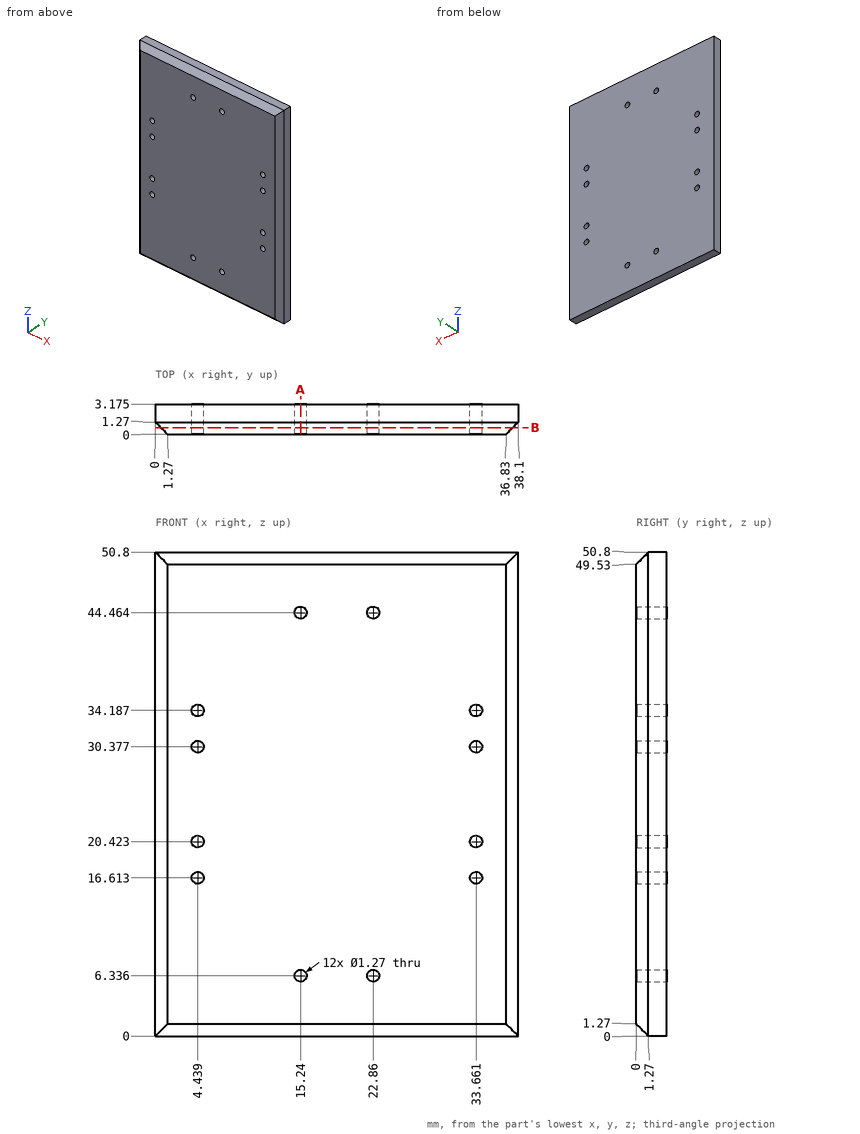
Geometry check sheet. Reference: drawing and pictorial views, mm from the part's lowest x, y, z. Give positions to 0.01 mm unless a question says otherwise; leave off trailing zeros. Write each loop counter-clockwise with the first axis right and the second up, starting at its lowest first coordinate (ties: lowest second). Pieces come first, ordered by that corner, then holes.
Item 1: Cross-section at B-B (y = 0.7). Count the separate pieces of the cut face and the enclosed holes in it, and give its area (3 significant figures).
Item 2: Scan lines: L1, parallel to X at y = 1.75, z = 30.5; L2, parallel to X at y = 0.2, z = 44 (1 decimal); L3, parallel to Z at x = 5, y = 1.55 (1 decimal). Record each from-to range of solid material in increasing order.
Item 3: Cross-section at A-A (x = 15.24). Enter the section's corners in (y, z) (1 decimal).
Item 4: Gauge pin test, flat end, axial feed: pin 1 (0.8 mm diameter, centred on x = 33.66, z = 16.61, fed in from +Y) (1 decimal). Record the tip position at first contact, or that the pin passes through.
Report:
1. separate pieces: 1
1. enclosed holes: 12
1. area: 1,820 mm2
2. L1: x = 0 to 3.82, 5.06 to 33.04, 34.28 to 38.1
2. L2: x = 1.1 to 14.8, 15.7 to 22.4, 23.3 to 37
2. L3: z = 0 to 16.3, 16.9 to 20.1, 20.7 to 30.1, 30.7 to 33.9, 34.5 to 50.8
3. outline: (0, 1.3) - (1.3, 0) - (3.2, 0) - (3.2, 5.7) - (0, 5.7) - close; (0, 7) - (3.2, 7) - (3.2, 43.8) - (0, 43.8) - close; (0, 45.1) - (3.2, 45.1) - (3.2, 50.8) - (1.3, 50.8) - (0, 49.5) - close
4. pin 1: passes through
